Can you work these out from the drawing? Everything is in mm from the part's minimum corner. A direction names the side the tool comes from. Coordinates: 2 decimals unless noted, no trailing zeros. Order: outer loops, then holes, each group sorted by start corner. A loop starts at its lowest first (then second) coordinate and runs counter-clockwise, first axis right, second up. Notation, with made-up numbers: (83.5, 64) - (129.5, 64) arc R34 ccw to (129.5, 100) - close; hole circle Ø8 at (85.25, 66.25). An arc over 180 degrees is marked (long way). Use CSV: the item, a comma, the result in double quotes. Start each with the question number.
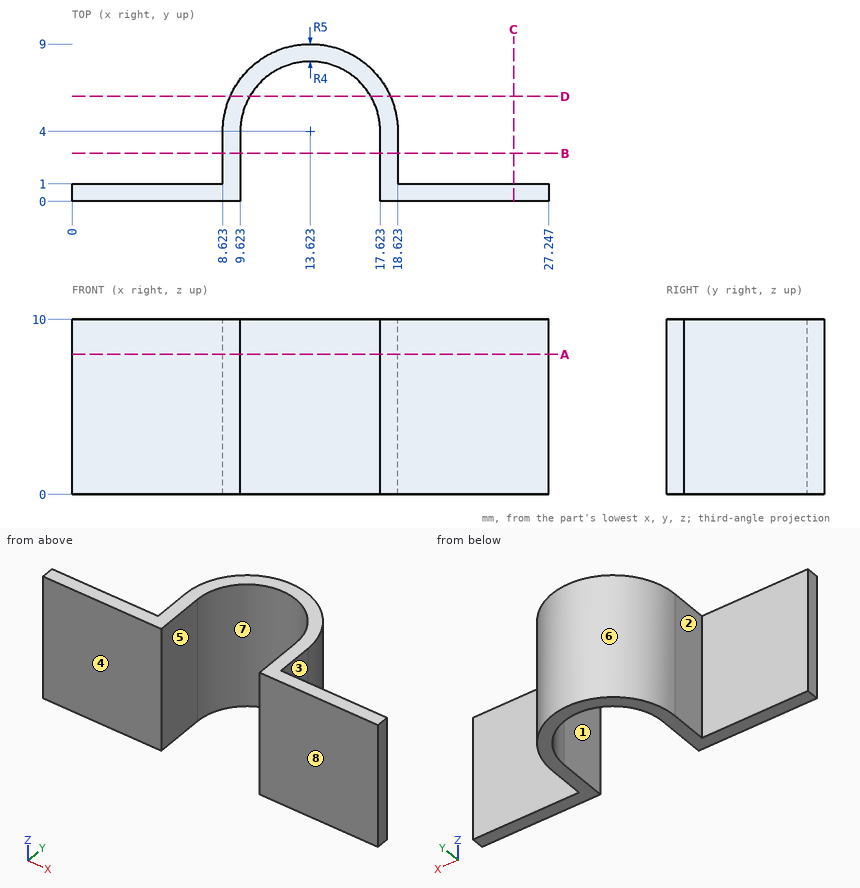
Item 1: Suppose I cut it at C-C on x = 25.25. Write out the boundary of the cut face in (y, z).
Item 2: For the marked faces 1, 2, 3 and 4, which set-ups out of +Z, -Z, +X, -X, +Y, -Y let a thin tool reach every point of the face, with its end or its side?
Item 3: Suppose I cut it at A-A on z = 8. Write out the boundary of the cut face in (x, y).
Item 4: We'd pull the mould along X, two halves only. Please class the marked faces 5, 6, 7 and 8: released by +X, released by -X, zero draft, split by the parting line, or undercut.
Item 5: For pin 1 Ø4 at (x, z) = (3.5, 8) entering from -Y; pin 2 Ø3 at (y, z) = (3, 6) entering from -X; pin 3 Ø2.5 at (y, z) = (3, 7) entering from +X; pin 4 Ø1 at (x, y) = (13.5, 5.5) entering from +Z, each with a flat end and sliding along its axis, tell me the tip position at first contact or that it passes through.
Item 6: Please list where these lines run through material, in increasing order: line 1 along X through (y, z) = (0.5, 0.5); line 2 along X through (y, z) = (4, 4); line 3 along Y through (x, z) = (7.25, 1). Write a range as from..to.
Item 7: Suppose I cut it at B-B on y = 2.75. Write out the boundary of the cut face in (x, z), then the cut area to 3 significant figures.
Item 8: Suppose I cut it at D-D on y = 6. Write out the boundary of the cut face in (x, z).
Here are the results:
1,outline,"(0, 0) - (1, 0) - (1, 10) - (0, 10) - close"
2,face 1,"+Z, -Z, -Y"
2,face 2,"+Z, -Z, -X, +Y"
2,face 3,"+Z, -Z, +X, +Y"
2,face 4,"+Z, -Z, +X, -X, -Y"
3,outline,"(0, 0) - (9.62, 0) - (9.62, 4) arc R4 cw to (17.62, 4) - (17.62, 0) - (27.25, 0) - (27.25, 1) - (18.62, 1) - (18.62, 4) arc R5 ccw to (8.62, 4) - (8.62, 1) - (0, 1) - close"
4,face 5,"undercut"
4,face 6,"split by the parting line"
4,face 7,"undercut"
4,face 8,"zero draft"
5,pin 1,"y = 0"
5,pin 2,"x = 8.62"
5,pin 3,"x = 18.62"
5,pin 4,"through"
6,line 1,"0..9.62, 17.62..27.25"
6,line 2,"8.62..9.62, 17.62..18.62"
6,line 3,"0..1"
7,outline,"(8.62, 0) - (9.62, 0) - (9.62, 10) - (8.62, 10) - close; (17.62, 0) - (18.62, 0) - (18.62, 10) - (17.62, 10) - close"
7,area,"20.0 mm^2"
8,outline,"(9.04, 0) - (10.16, 0) - (10.16, 10) - (9.04, 10) - close; (17.09, 0) - (18.21, 0) - (18.21, 10) - (17.09, 10) - close"
